Check sheet for the modelled part. Datum: model origin and axes. Units: mm. Face numbers are marked on the shaded views. A direction names the side the tool comes from. Round coordinates to 2 decimals unless told otherwise and drop trailing zeros. Order: outer loops, then holes, each group sorted by start corner. A loop starts at its lowest first (then second) coordinate and runs counter-clockwise, first axis right, second up. Notation, with made-up numbers: (58, 59.5) -> (117, 59.5) arc R22 cw to (117, 87.5) -> close; hole circle Ø1 at (-31.5, 78). An arc over 180 degrees is marked (long way). Use CSV: the item, a comma, the result in double quotes.
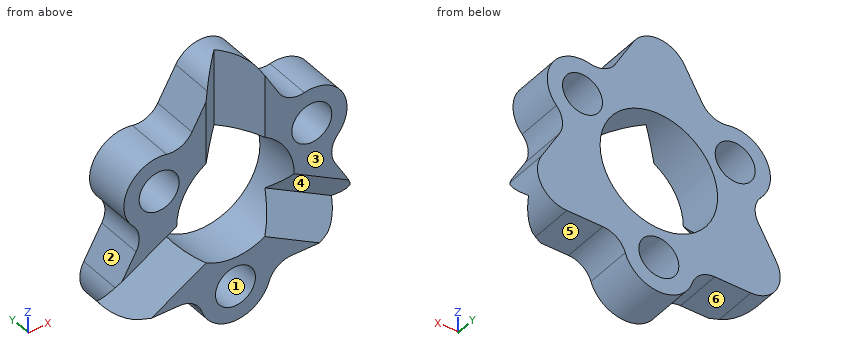
```python
from build123d import *

# Parameters (mm, degrees)
SKETCH1_R         = 5
EXTRUDE1_DEPTH    = 4
CIRPATTERN2_COUNT = 3
EXTRUDE4_START    = 4.45086
EXTRUDE4_DEPTH    = 7.205259
EXTRUDE5_START    = 4.330127
EXTRUDE5_DEPTH    = 7.205258
EXTRUDE6_START    = 4.330127
EXTRUDE6_DEPTH    = 7.205258


with BuildPart() as part:
    # Sketch1 → Extrude1 (new body)
    with BuildSketch(Plane(origin=(0, 0, 0), x_dir=(1, 0, 0), z_dir=(0, 1, 0))):
        with BuildLine():
            Line((-3.89089061, 3.146959138), (-2.360502052, 0.4962484))
            ThreePointArc((-2.360502052, 0.4962484), (-2.104118872, -0.718531203), (-2.613989574, -1.850544314))
            ThreePointArc((-2.613989574, -1.850544314), (-2.994220859, -5.370733384), (0.244467944, -6.801537968))
            ThreePointArc((0.244467944, -6.801537968), (1.479755407, -6.925983542), (2.403593813, -7.75540769))
            Line((2.403593813, -7.75540769), (3.933982371, -10.406118428))
            ThreePointArc((3.933982371, -10.406118428), (6.099045881, -11.656118428), (8.26410939, -10.406118428))
            Line((8.26410939, -10.406118428), (9.794497948, -7.75540769))
            ThreePointArc((9.794497948, -7.75540769), (10.718336354, -6.925983542), (11.953623817, -6.801537968))
            ThreePointArc((11.953623817, -6.801537968), (15.192312621, -5.370733384), (14.812081336, -1.850544314))
            ThreePointArc((14.812081336, -1.850544314), (14.302210633, -0.718531203), (14.558593813, 0.4962484))
            Line((14.558593813, 0.4962484), (16.088982371, 3.146959138))
            ThreePointArc((16.088982371, 3.146959138), (16.088982371, 5.646959138), (13.923918862, 6.896959138))
            Line((13.923918862, 6.896959138), (10.863141746, 6.896959138))
            ThreePointArc((10.863141746, 6.896959138), (9.68292016, 7.282314592), (8.9575034, 8.289882129))
            ThreePointArc((8.9575034, 8.289882129), (6.099045881, 10.379266616), (3.240588362, 8.289882129))
            ThreePointArc((3.240588362, 8.289882129), (2.515171602, 7.282314592), (1.334950016, 6.896959138))
            Line((1.334950016, 6.896959138), (-1.7258271, 6.896959138))
            ThreePointArc((-1.7258271, 6.896959138), (-3.89089061, 5.646959138), (-3.89089061, 3.146959138))
        make_face()
        with Locations((6.099045881, -0.120733384)):
            Circle(SKETCH1_R, mode=Mode.SUBTRACT)
    extrude(amount=EXTRUDE1_DEPTH)

    # Sketch6 → M3 Clearance Hole1 (revolve, cut)
    with BuildSketch(Plane(origin=(-0.396144648, 4, 3.870733384), x_dir=(0, 0, 1), z_dir=(1, 0, 0))):
        Polygon((0, 0), (0, 11.021463052), (1.7, 10), (1.7, 0), align=None)
    m3_clearance_hole1 = revolve(axis=Axis((-0.396144648, 10.35, 3.870733384), (0, -1, 0)), mode=Mode.SUBTRACT)

    # CirPattern2: M3 Clearance Hole1 ×3 about axis
    cirpattern2_axis = Axis((6.099045881, 0, 0.120733384), (0, 1, 0))
    for i in range(1, CIRPATTERN2_COUNT):
        add(m3_clearance_hole1.rotate(cirpattern2_axis, i * 360 / CIRPATTERN2_COUNT), mode=Mode.SUBTRACT)

    # GrooveSketch → Extrude4 (cut)
    with BuildSketch(Plane.XY.offset(EXTRUDE4_START)):
        Polygon((34.668922444, -26.069876563), (8.599045881, 0), (6.099045881, 2.5), (3.599045881, 0), (-22.470830682, -26.069876563), (-22.470830682, -99.806622573), (34.668922444, -99.806622573), align=None)
    extrude(amount=EXTRUDE4_DEPTH, mode=Mode.SUBTRACT)

    # Sketch9 → Extrude5 (cut)
    with BuildSketch(Plane(origin=(4.6265635, 0, 2.671147682), x_dir=(-0.5, 0, 0.866025404), z_dir=(-0.866025404, 0, -0.5)).offset(EXTRUDE5_START)):
        Polygon((32.223222882, -32.668187644), (-0.444964763, 0), (-2.944964763, 2.5), (-5.444964763, 0), (-38.113152407, -32.668187644), (-38.113152407, -125.067775694), (32.223222882, -125.067775694), align=None)
    extrude(amount=EXTRUDE5_DEPTH, mode=Mode.SUBTRACT)

    # Sketch10 → Extrude6 (cut)
    with BuildSketch(Plane(origin=(4.522005322, 0, -2.61078099), x_dir=(-0.5, 0, -0.866025404), z_dir=(0.866025404, 0, -0.5)).offset(EXTRUDE6_START)):
        Polygon((32.014106526, -32.668187644), (-0.654081118, 0), (-3.154081118, 2.5), (-5.654081118, 0), (-38.322268763, -32.668187644), (-38.322268763, -125.067775694), (32.014106526, -125.067775694), align=None)
    extrude(amount=EXTRUDE6_DEPTH, mode=Mode.SUBTRACT)


solid = part.part
```
Q1. Mould release check, pull along X, two halves, no side actions. Record for the marked faces 1, 2 and 3: pulls with the +X half, pulls with the -X half, needs draft (parallel to the pull), parting line crosses it, or undercut.
Result sheet:
face 1,"undercut"
face 2,"pulls with the -X half"
face 3,"needs draft"
Q2. Sectioned sample at C-C, the plane x = -3. Enter the section's corners in (y, z).
Result sheet:
outline,"(0, -2.25) -> (2.5, -5.13) -> (1.27, -6.55) -> (4, -6.55) -> (4, -1.6) -> (0, -1.6) -> close; (0, 2.38) -> (4, 2.38) -> (4, 5.36) -> (0, 5.36) -> close"
Q3. Access from +Z, -Z, +X, -X, +Y, -Y to the whole of each face (thin tool, end or side, straight path). Record for the marked faces 4, 5 and 6.
Result sheet:
face 4,"-Y"
face 5,"-Z, +X, +Y, -Y"
face 6,"-Z, -X, +Y, -Y"
Q4. Sectioned sample at A-A, the plane y = 1.65. State how many separate pieces and enclosed holes the cut face has, then the cut area to 3 significant figures.
Result sheet:
separate pieces,"3"
enclosed holes,"3"
area,"158 mm^2"
Q5. Go/stop test with flat-tipped pins: pin 1 (2 mm diameter, centred on y = 1, z = -7.5, fed in from +X); pin 2 (0.9 mm diameter, centred on x = 12, y = 2.5, fed in from -Z); pin 3 (1 mm diameter, centred on x = 2, y = 3, fed in from +Z). Record where each tip stops, or that it passes through.
Result sheet:
pin 1,"stops at x = 15.21"
pin 2,"stops at z = -6.9"
pin 3,"stops at z = 7.92"
Q6. Sectioned sample at B-B, the plane z = -7.25. Enter the section's corners in (x, y).
Result sheet:
outline,"(2.47, 0) -> (4.4, 0) -> (4.4, 4) -> (2.47, 4) -> close; (7.79, 0) -> (9.73, 0) -> (9.73, 4) -> (7.79, 4) -> close"
Q7. Sectioned sample at D-D, the plane y = 2.8. Enter the section's corners in (x, z).
Result sheet:
outline,"(-3.89, -3.15) arc R2.5 ccw to (-1.73, -6.9) -> (1.33, -6.9) arc R2 cw to (3.24, -8.29) arc R3 ccw to (8.96, -8.29) arc R2 cw to (10.86, -6.9) -> (13.92, -6.9) arc R2.5 ccw to (16.09, -3.15) -> (14.56, -0.5) arc R2 cw to (14.81, 1.85) arc R3 ccw to (11.95, 6.8) arc R2 cw to (9.79, 7.76) -> (8.26, 10.41) arc R2.5 ccw to (3.93, 10.41) -> (2.4, 7.76) arc R2 cw to (0.24, 6.8) arc R3 ccw to (-2.61, 1.85) arc R2 cw to (-2.36, -0.5) -> close; hole circle Ø3.4 at (-0.4, 3.87); hole circle Ø10 at (6.1, 0.12); hole circle Ø3.4 at (6.1, -7.38); hole circle Ø3.4 at (12.59, 3.87)"
Q8. Scan lines: L1, parallel to Z at x = 5.25, y = 1.8; L2, parallel to X at y = 3.05, z = 4.25; L3, parallel to X at y = 2.35, z = 4. Record each from-to range of solid material in increasing order.
Result sheet:
L1,"z = -10.26 to -8.85, -5.91 to -4.81, 5.05 to 11.51"
L2,"x = -3.37 to -2.05, 1.26 to 3.28, 8.92 to 10.94, 14.25 to 15.57"
L3,"x = -3.39 to -2.09, 1.3 to 2.94, 9.25 to 10.9, 14.29 to 15.59"
